Could you check a few things on this model? Use its own coordinates, in mm. A direction names the side the tool comes from. Coordinates: 2 decimals unless noted, no trailing zeros. Order: outer loops, then holes, each group sorted by start corner. A loop starts at its lowest first (then second) coordinate and runs counter-clockwise, first axis right, second up. Notation, with made-up numbers: (85, 43) - (126, 43) arc R26 ccw to (126, 81) - close; hole circle Ø9 at (20.25, 9). An arc over 180 degrees is marked (long way). One line per item, written item: value.
from build123d import *

# Parameters (mm, degrees)
BOSS_EXTRUDE1_DEPTH     = 50
SKETCH5_W               = 40
SKETCH5_H               = 50
CUT_EXTRUDE4_DEPTH      = 10
SKETCH6_R               = 7.5
CUT_EXTRUDE5_DEPTH      = 15
CUT_EXTRUDE6_DEPTH      = 65.007812023
CUT_EXTRUDE6_DEPTH_BACK = 65.007812023
SKETCH7_R               = 2.8
SKETCH8_R               = 8.913017029
SKETCH8_R_2             = 2.2
CUT_EXTRUDE7_DEPTH      = 10
SKETCH12_R              = 35
CUT_EXTRUDE8_DEPTH      = 6


with BuildPart() as part:
    # Sketch1 → Boss-Extrude1 (new body)
    with BuildSketch(Plane.XY):
        with BuildLine():
            Line((34, 6), (-34, 6))
            ThreePointArc((-34, 6), (-29.606601718, 16.606601718), (-19, 21))
            Line((-19, 21), (19, 21))
            ThreePointArc((19, 21), (29.606601718, 16.606601718), (34, 6))
        make_face()
    extrude(amount=BOSS_EXTRUDE1_DEPTH)

    # Sketch5 → Cut-Extrude4 (cut)
    with BuildSketch(Plane.XZ.offset(-6)):
        with Locations((0, 25)):
            Rectangle(SKETCH5_W, SKETCH5_H)
    extrude(amount=-CUT_EXTRUDE4_DEPTH, mode=Mode.SUBTRACT)

    # Sketch6 → Cut-Extrude5 (cut)
    with BuildSketch(Plane(origin=(0, 21, 0), x_dir=(1, 0, 0), z_dir=(0, 1, 0))):
        with Locations(Location((0, -25, 0), (0, 0, 270))):
            Circle(SKETCH6_R)
    extrude(amount=-CUT_EXTRUDE5_DEPTH, mode=Mode.SUBTRACT)

    # Sketch7 → Cut-Extrude6 (cut, two sides: drawn at the far end of the back side and taken through both)
    with BuildSketch(Plane.XY.offset(50).offset(-CUT_EXTRUDE6_DEPTH_BACK)):
        with Locations((-26, 11)):
            Circle(SKETCH7_R)
        with Locations((26, 11)):
            Circle(SKETCH7_R)
    extrude(amount=CUT_EXTRUDE6_DEPTH + CUT_EXTRUDE6_DEPTH_BACK, mode=Mode.SUBTRACT)

    # Sketch8 → Cut-Extrude7 (cut)
    with BuildSketch(Plane(origin=(0, 21, 0), x_dir=(1, 0, 0), z_dir=(0, 1, 0))):
        with Locations(Location((0, -25, 0), (0, 0, 180))):
            Circle(SKETCH8_R)
        with Locations(Location((10.606601718, -14.393398282, 0), (0, 0, 180))):
            Circle(SKETCH8_R_2)
        with Locations(Location((15.556349186, -9.443650814, 0), (0, 0, 180))):
            Circle(SKETCH8_R_2)
        with Locations(Location((-10.606601718, -14.393398282, 0), (0, 0, 180))):
            Circle(SKETCH8_R_2)
        with Locations(Location((-15.556349186, -9.443650814, 0), (0, 0, 180))):
            Circle(SKETCH8_R_2)
        with Locations(Location((-10.606601718, -35.606601718, 0), (0, 0, 180))):
            Circle(SKETCH8_R_2)
        with Locations(Location((-15.556349186, -40.556349186, 0), (0, 0, 180))):
            Circle(SKETCH8_R_2)
        with Locations(Location((10.606601718, -35.606601718, 0), (0, 0, 180))):
            Circle(SKETCH8_R_2)
        with Locations(Location((15.556349186, -40.556349186, 0), (0, 0, 180))):
            Circle(SKETCH8_R_2)
    extrude(amount=-CUT_EXTRUDE7_DEPTH, mode=Mode.SUBTRACT)

    # Sweep2: sweep along a path in Sketch11
    with BuildLine(Plane(origin=(0, 0, 0), x_dir=(-1, 0, 0), z_dir=(0, 0, -1))) as sweep2_path:
        ThreePointArc((-34, 6), (-29.606601718, 16.606601718), (-19, 21))
        Line((-19, 21), (19, 21))
        ThreePointArc((19, 21), (29.606601718, 16.606601718), (34, 6))
    # Sketch9 → Sweep2 (sweep)
    with BuildSketch(Plane.XZ.offset(-6)):
        Polygon((34, 0), (36, 2), (36, 9.5), (38, 11.5), (38, 17), (40, 19), (40, 31), (38, 33), (38, 38.5), (36, 40.5), (36, 48), (34, 50), align=None)
    sweep(path=sweep2_path.line)

    # Sketch12 → Cut-Extrude8 (cut)
    with BuildSketch(Plane(origin=(0, 27, 0), x_dir=(1, 0, 0), z_dir=(0, 1, 0))):
        with Locations((0, -25)):
            Circle(SKETCH12_R)
    extrude(amount=-CUT_EXTRUDE8_DEPTH, mode=Mode.SUBTRACT)


solid = part.part
Item 1: I'm going to push flat-ended pins straight in: pin 1 Ø8 at (y, z) = (9, 13) entering from +X; pin 2 Ø5 at (x, z) = (15.56, 9.44) entering from -Y; pin 3 Ø1 at (x, z) = (-9, 45) entering from +Y; pin 4 Ø2.5 at (x, z) = (10.61, 14.39) entering from +Y. Where does each tip first touch, or does it pass through?
Conclusion:
pin 1: x = 38
pin 2: y = 16
pin 3: y = 21
pin 4: through
Item 2: I want a section at C-C on y = 11. Give the number of separate pieces and of enclosed holes in the cut face, then the cut area to 3 significant figures.
Conclusion:
separate pieces: 4
enclosed holes: 0
area: 1,140 mm²
Item 3: If I drill on probe 1 along Y at (x, z) = (-26, 40); probe 2 along X at (y, z) = (12.75, 12.5); probe 3 along X at (y, z) = (8.5, 35.5), over which ranges is the centre line in solid material (lowest first)?
Conclusion:
probe 1: 6 to 8.2, 13.8 to 21
probe 2: -36.76 to -28.19, -23.81 to -20, 20 to 23.81, 28.19 to 36.76
probe 3: -37.83 to -27.26, -24.74 to -20, 20 to 24.74, 27.26 to 37.83
Item 4: I want a section at A-A on z = 25. Please give me the cut outline in (x, y), then the cut area to 3 significant figures.
Conclusion:
outline: (-40, 6) - (-20, 6) - (-20, 16) - (-8.91, 16) - (-8.91, 21) - (-33.7, 21) arc R21 ccw to start; (8.91, 16) - (20, 16) - (20, 6) - (40, 6) arc R21 ccw to (33.7, 21) - (8.91, 21) - close; hole circle Ø5.6 at (-26, 11); hole circle Ø5.6 at (26, 11)
area: 603 mm²
Item 5: Thinking about a two-plate mould opening in Y: for faces 5 (the face through (23.2, 11.1, 24.6)), 6 (the face through (-17.655, 18.535, 10.104)), 7 (the face through (31.645, 14.648, 49.681)), which applies, pulls with the +Y half, pulls with the -Y half, needs draft (parallel to the pull), parting line crosses it, or undercut?
Conclusion:
face 5: undercut
face 6: needs draft
face 7: pulls with the +Y half
Item 6: For faces 1 (the face through (33.467, 14.929, 5.802)), 2 (the face through (38.405, 14.027, 25.084)), 3 (the face through (20, 11, 25)), 4 (the face through (33.467, 14.929, 44.302)), which set-ups out of +Z, -Z, +X, -X, +Y, -Y let a thin tool reach every point of the face, with its end or its side?
Conclusion:
face 1: -Z, +X, +Y
face 2: +Z, -Z, +X, +Y
face 3: +Z, -Z, -Y
face 4: +Z, +X, +Y
Item 7: I want a section at B-B on x = 0. Please give me the cut outline in (y, z), then the cut area to 3 significant figures.
Conclusion:
outline: (16, 0) - (21, 0) - (21, 16.09) - (16, 16.09) - close; (16, 33.91) - (21, 33.91) - (21, 50) - (16, 50) - close
area: 161 mm²
